For this review, take the finished solid that the model builds, in its own axes (mm). A direction names the side the tool comes from. Coordinates: 2 decimals unless noted, no trailing zeros. Loops run counter-clockwise (first coordinate to the right, second up) from the corner with the lowest first, then second, coordinate; pieces in that order, holes last. Notation, with made-up numbers: M -34,20 L -9,20 A18 cw -9,24 Z; hole C -0.75,31 d4. An arc over 180 degrees is marked long. Put each result on its own line as item: value.
```python
from build123d import *

# Parameters (mm, degrees)
SKETCH1_R           = 1.388229101
SKETCH1_R_2         = 1.314910669
SKETCH1_R_3         = 1.856429035
SKETCH1_R_4         = 2
SKETCH1_R_5         = 1.65
SKETCH1_R_6         = 1.483383261
SKETCH1_R_7         = 1.248623853
SKETCH1_R_8         = 1.255629307
SKETCH1_R_9         = 7
SKETCH1_R_10        = 1.53911217
BOSS_EXTRUDE1_DEPTH = 1.5875
SKETCH4_W           = 66.272407177
SKETCH4_H           = 27.800260981
CUT_EXTRUDE2_DEPTH  = 20
FILLET3_R           = 10
FILLET4_R           = 10
BOSS_EXTRUDE3_START = -1.5875
BOSS_EXTRUDE3_DEPTH = 1.5875
SKETCH7_R           = 7
CUT_EXTRUDE3_DEPTH  = 1.5875
SKETCH8_W           = 100.106183873
SKETCH8_H           = 60.21728362
CUT_EXTRUDE4_DEPTH  = 35
FILLET5_R           = 10


with BuildPart() as part:
    # Sketch1 → Boss-Extrude1 (new body)
    with BuildSketch(Plane(origin=(0, 0, 0), x_dir=(1, 0, 0), z_dir=(0, 1, 0))):
        with BuildLine():
            Line((42.32729629, 228.6), (10.454309325, 228.6))
            Line((10.454309325, 228.6), (0, 135.362739137))
            Line((0, 135.362739137), (0, 0))
            Line((0, 0), (24.327009544, 0))
            Line((24.327009544, 0), (50.8, 0))
            Line((50.8, 0), (50.8, 64.87909603))
            Line((50.8, 64.87909603), (50.8, 87.423477361))
            Line((50.8, 87.423477361), (50.8, 98.200996728))
            ThreePointArc((50.8, 98.200996728), (50.4, 101.000996728), (50.8, 103.800996728))
            Line((50.8, 103.800996728), (50.8, 104.488200565))
            Line((50.8, 104.488200565), (50.8, 120.619222808))
            Line((50.8, 120.619222808), (50.8, 135.362739137))
            Line((50.8, 135.362739137), (42.32729629, 228.6))
        make_face()
        with Locations(Location((6.335590122, 44.288799513, 0), (0, 0, 270))):
            Circle(SKETCH1_R, mode=Mode.SUBTRACT)
        with Locations(Location((4.659546827, 82.793173401, 0), (0, 0, 270))):
            Circle(SKETCH1_R_2, mode=Mode.SUBTRACT)
        with Locations(Location((16.389129236, 58.804246097, 0), (0, 0, 270))):
            Circle(SKETCH1_R_3, mode=Mode.SUBTRACT)
        with Locations(Location((16.113249369, 74.801867492, 0), (0, 0, 270))):
            Circle(SKETCH1_R_4, mode=Mode.SUBTRACT)
        with Locations(Location((32.386750631, 59.080125965, 0), (0, 0, 270))):
            Circle(SKETCH1_R_5, mode=Mode.SUBTRACT)
        with Locations(Location((32.110870764, 75.07774736, 0), (0, 0, 270))):
            Circle(SKETCH1_R_4, mode=Mode.SUBTRACT)
        with BuildLine():
            Line((34.925740903, 92.78493524), (9.492033273, 92.78493524))
            ThreePointArc((9.492033273, 92.78493524), (6.992033273, 95.28493524), (9.492033273, 97.78493524))
            Line((9.492033273, 97.78493524), (34.925740903, 97.78493524))
            ThreePointArc((34.925740903, 97.78493524), (36.693507856, 97.052702193), (37.425740903, 95.28493524))
            ThreePointArc((37.425740903, 95.28493524), (36.693507856, 93.517168287), (34.925740903, 92.78493524))
        make_face(mode=Mode.SUBTRACT)
        with BuildLine():
            Line((34.925740903, 105.90993524), (9.492033273, 105.90993524))
            ThreePointArc((9.492033273, 105.90993524), (6.492033273, 108.90993524), (9.492033273, 111.90993524))
            Line((9.492033273, 111.90993524), (34.925740903, 111.90993524))
            ThreePointArc((34.925740903, 111.90993524), (37.047061246, 111.031255584), (37.925740903, 108.90993524))
            ThreePointArc((37.925740903, 108.90993524), (37.047061246, 106.788614896), (34.925740903, 105.90993524))
        make_face(mode=Mode.SUBTRACT)
        with Locations(Location((43.447673368, 42.868436544, 0), (0, 0, 270))):
            Circle(SKETCH1_R_6, mode=Mode.SUBTRACT)
        with Locations(Location((48.400988852, 71.551011715, 0), (0, 0, 270))):
            Circle(SKETCH1_R_7, mode=Mode.SUBTRACT)
        with Locations(Location((5.88467603, 135.103145298, 0), (0, 0, 270))):
            Circle(SKETCH1_R_8, mode=Mode.SUBTRACT)
        with BuildLine():
            Line((35.509675341, 119.784935244), (9.492033273, 119.784935244))
            ThreePointArc((9.492033273, 119.784935244), (7.026609419, 122.250359097), (9.492033273, 124.71578295))
            Line((9.492033273, 124.71578295), (35.509675341, 124.71578295))
            ThreePointArc((35.509675341, 124.71578295), (37.252993266, 123.993677022), (37.975099194, 122.250359097))
            ThreePointArc((37.975099194, 122.250359097), (37.252993266, 120.507041172), (35.509675341, 119.784935244))
        make_face(mode=Mode.SUBTRACT)
        with Locations(Location((29.504213454, 189.557234372, 0), (0, 0, 270))):
            Circle(SKETCH1_R_9, mode=Mode.SUBTRACT)
        with Locations(Location((45.747747887, 129.863467374, 0), (0, 0, 270))):
            Circle(SKETCH1_R_10, mode=Mode.SUBTRACT)
    extrude(amount=BOSS_EXTRUDE1_DEPTH)

    # Sketch4 → Cut-Extrude2 (cut)
    with BuildSketch(Plane(origin=(0, 0, -228.6), x_dir=(-1, 0, 0), z_dir=(0, 0, -1))):
        with Locations((-28.174690156, -1.980940155)):
            Rectangle(SKETCH4_W, SKETCH4_H)
    extrude(amount=-CUT_EXTRUDE2_DEPTH, mode=Mode.SUBTRACT)

    # Fillet3
    fillet3_edges = [part.edges().sort_by_distance(p)[0] for p in [
        (44.144746445, 0.79375, -208.6),
    ]]
    fillet(fillet3_edges, radius=FILLET3_R)

    # Fillet4
    fillet4_edges = [part.edges().sort_by_distance(p)[0] for p in [
        (50.8, 0.79375, 0),
        (0, 0.79375, 0),
        (8.211791854, 0.79375, -208.6),
    ]]
    fillet(fillet4_edges, radius=FILLET4_R)

    # Sketch6 → Boss-Extrude3 (add)
    with BuildSketch(Plane(origin=(0, 1.5875, 0), x_dir=(1, 0, 0), z_dir=(0, 1, 0)).offset(BOSS_EXTRUDE3_START)):
        with BuildLine():
            Line((50.8, 135.362739137), (50.8, 103.800996728))
            ThreePointArc((50.8, 103.800996728), (50.4, 101.000996728), (50.8, 98.200996728))
            Line((50.8, 98.200996728), (50.8, 61.124243317))
            Line((50.8, 61.124243317), (69.258211507, 96.360728536))
            ThreePointArc((69.258211507, 96.360728536), (70.393157133, 101.370875786), (68.890940865, 106.283413148))
            Line((68.890940865, 106.283413148), (50.8, 135.362739137))
        make_face()
    extrude(amount=BOSS_EXTRUDE3_DEPTH)

    # Sketch7 → Cut-Extrude3 (cut)
    with BuildSketch(Plane(origin=(0, 1.5875, 0), x_dir=(1, 0, 0), z_dir=(0, 1, 0))):
        with Locations(Location((60.4, 101.000996728, 0), (0, 0, 270))):
            Circle(SKETCH7_R)
    extrude(amount=-CUT_EXTRUDE3_DEPTH, mode=Mode.SUBTRACT)

    # Sketch8 → Cut-Extrude4 (cut)
    with BuildSketch(Plane.XY):
        with Locations((28.455154517, 1.704032249)):
            Rectangle(SKETCH8_W, SKETCH8_H)
    extrude(amount=-CUT_EXTRUDE4_DEPTH, mode=Mode.SUBTRACT)

    # Fillet5
    fillet5_edges = [part.edges().sort_by_distance(p)[0] for p in [
        (0, 0.79375, -35),
        (50.8, 0.79375, -35),
    ]]
    fillet(fillet5_edges, radius=FILLET5_R)


solid = part.part
```
(1) Add section A-A (x = 62.5). Write out the cut boundary in (y, z), plus the area to 3 significant figures.
Determined:
outline: M 0,-116.56 L 1.59,-116.56 L 1.59,-107.68 L 0,-107.68 Z; M 0,-94.32 L 1.59,-94.32 L 1.59,-83.46 L 0,-83.46 Z
area: 31.3 mm^2
(2) Add section B-B (z = -48). Write out the cut boundary in (x, y), plus the area to 3 significant figures.
Determined:
outline: M 0,0 L 50.8,0 L 50.8,1.59 L 0,1.59 Z
area: 80.6 mm^2
(3) Add section C-C (y = 0.95). State how many separate pieces and enclosed holes the cut face has, plus the area to 3 significant figures.
Determined:
separate pieces: 1
enclosed holes: 15
area: 8,110 mm^2
(4) Wall thickness on line 1 along Z through (x, y) = (21.5, 0.85); line 2 along Z through (x, y) = (15, 0.25); line 3 along X through (y, z) = (0.7, -74): over which ranges is each line inside the solid? List them lowest first. Write a range as [from, to].
Determined:
line 1: z = [-208.6, -124.72], [-119.78, -111.91], [-105.91, -97.78], [-92.78, -35]
line 2: z = [-208.37, -124.72], [-119.78, -111.91], [-105.91, -97.78], [-92.78, -76.46], [-73.14, -60.04], [-57.57, -35]
line 3: x = [0, 14.28], [17.95, 30.43], [33.8, 57.54]
(5) For pin 1 (12 mm diameter, centred on x = 60.5, z = -86.5, fed in from -Y), flat-tipped, find the tip position at first contact; note if it passes through.
Determined:
pin 1: stops at y = 0
(6) Add section D-D (z = -139). Write out the cut boundary in (x, y), plus the area to 3 significant figures.
Determined:
outline: M 0.41,0 L 50.47,0 L 50.47,1.59 L 0.41,1.59 Z
area: 79.5 mm^2
(7) Tool access review of faces 1 (the cylindrical face through (6.493, 0.783, -108.844)), 2 (the flat face through (27, 0, -104)): name each direction out of +Z, -Z, +X, -X, +Y, -Y from which nothing blocks a thin tool from reaching the whole face with its end or side.
Determined:
face 1: +Y, -Y
face 2: +Z, -Z, +X, -X, -Y
(8) Draft analysis for pull direction X (two halves, no side actions). For faces 3 (the cylindrical face through (29.81, 0.78, -196.55)), 4 (the cylindrical face through (41.832, 0.783, -205.914)), 5 (the flat face through (3.66, 0.78, -167.99)), 6 (the cylindrical face through (16.2, 0.8, -76.8)), state which applies: +X half, -X half, draft (parallel to the pull), parting line (faces both ways), or undercut.
Determined:
face 3: undercut
face 4: +X half
face 5: -X half
face 6: undercut
